```python
from build123d import *

# Parameters (mm, degrees)
F0_R            = 10
F0_R_2          = 7.5
F1_DEPTH        = 2
F3_DEPTH        = 25
F3_COPIES_COUNT = 3
F4_R            = 1
F5_DEPTH        = 25
F5_COPIES_COUNT = 3


# Not quite as in the source:
# - a pattern or mirror of a feature is missing from the dataset's text; its kind, count and spacing are read off the source's solid


with BuildPart() as f1:
    # F0 (on Front) → F1 (new body)
    with BuildSketch(Plane.XZ):
        Circle(F0_R)
        Circle(F0_R_2, mode=Mode.SUBTRACT)
    extrude(amount=F1_DEPTH)

    # F2 (on Top) → F3 (cut)
    with BuildSketch(Plane.XY):
        Polygon((-1.2, 0), (0, -1.2), (1.2, 0), align=None)
    f3 = extrude(amount=-F3_DEPTH, mode=Mode.SUBTRACT)

    # F3_copies: F3 ×3 about axis
    f3_copies_axis = Axis((0, 0, 0), (0, 1, 0))
    for i in range(1, F3_COPIES_COUNT):
        add(f3.rotate(f3_copies_axis, i * 360 / F3_COPIES_COUNT), mode=Mode.SUBTRACT)

    # F4 (on Front) → F5 (join)
    with BuildSketch(Plane.XZ):
        with Locations((0, 8.75)):
            Circle(F4_R)
    f5 = extrude(amount=-F5_DEPTH)

    # F5_copies: F5 ×3 about axis
    f5_copies_axis = Axis((0, 0, 0), (0, 1, 0))
    for i in range(1, F5_COPIES_COUNT):
        add(f5.rotate(f5_copies_axis, i * 360 / F5_COPIES_COUNT))


solid = f1.part
```
Work out the finished part from the listing and answer in its coordinate system (mm). A direction names the side the tool comes from. Coordinates: 2 decimals unless noted, no trailing zeros. Write each loop counter-clockwise with the first axis right and the second up, starting at its lowest first coordinate (ties: lowest second). Pieces come first, ordered by that corner, then holes.
Q1. Find the intervals of material crossed by line 1 (X direction, y = -0.75, z = 0); line 2 (Z direction, x = 0, y = -0.65); line 3 (X direction, y = -0.75, z = -5.25), in increasing order.
Q2. Which of the six approach directions +Z, -Z, +X, -X, +Y, -Y give full straight-line access (tool end or side, diameter ignored) to faces 1 (the face through (7.82, -0.59, 3.81)), 2 (the face through (-0.6, -0.6, -8.7)), 3 (the face through (-8, 25, -4))?
Q3. Each of these flat-tipped pins is pushed along its axis until it touches: pin 1 Ø8 at (x, y) = (6, 13.5) entering from +Z (3 decimals); pin 2 Ø6 at (y, z) = (19, 5.5) entering from -X; pin 3 Ø1 at (x, y) = (-6.5, 19.5) entering from -Z. Where does it stop, or does it pass through?
Q4. A cutting plane is placed at D-D, the plane z = 8.75. Give the vertices of the cut face in (x, y), then the cut area to 3 significant figures.
Q5. Determine the mould class of faces 4 (the face through (8, 25, -4)), 5 (the face through (-7.816, -0.608, 3.829)), 6 (the face through (8.53, 12.32, -4.07)), 7 (the face through (-2.17, -0.99, -9.76)) for opening direction X: released by +X, released by -X, zero draft, split by the parting line, or undercut.
Q6. A cutting plane is placed at B-B, the plane x = 4. Give the vertices of the cut face in (y, z), then the cut area to 3 significant figures.
Q7. A cutting plane is placed at C-C, the plane y = 21. Give the vertices of the cut face in (x, z) (3 decimals).
Q8. A cutting plane is placed at A-A, the plane z = 0. Give the vertices of the cut face in (x, y).
Findings below:
1. line 1: x = -10 to -7.5, 7.5 to 10
1. line 2: z = 7.5 to 10
1. line 3: x = -8.51 to -5.36, 5.36 to 8.51
2. face 1: +Y
2. face 2: -Z, +Y
2. face 3: +Z, -Z, +X, -X, +Y
3. pin 1: stops at z = -3.375
3. pin 2: stops at x = -0.97
3. pin 3: stops at z = -5.19
4. outline: (-4.84, -2) - (4.84, -2) - (4.84, 0) - (1, 0) - (1, 25) - (-1, 25) - (-1, 0) - (-4.84, 0) - close
4. area: 69.4 mm2
5. face 4: zero draft
5. face 5: undercut
5. face 6: undercut
5. face 7: split by the parting line
6. outline: (-2, -9.17) - (0, -9.17) - (0, -6.34) - (-2, -6.34) - close; (-2, 6.34) - (0, 6.34) - (0, 9.17) - (-2, 9.17) - close
6. area: 11.3 mm2
7. outline: circle Ø2 at (-7.578, -4.375); circle Ø2 at (0, 8.75); circle Ø2 at (7.578, -4.375)
8. outline: (-10, -2) - (-7.5, -2) - (-7.5, 0) - (-10, 0) - close; (7.5, -2) - (10, -2) - (10, 0) - (7.5, 0) - close
